Verification items for the finished model (mm, model axes). A direction names the side the tool comes from. Coordinates: 2 decimals unless noted, no trailing zeros. Order: outer loops, then holes, each group sorted by start corner. A loop starts at its lowest first (then second) coordinate and runs counter-clockwise, first axis right, second up. Notation, with made-up numbers: M -39.5,65.25 L -11.5,65.25 A6 ccw -11.5,73.25 Z; hole C 65,-16.75 d7. An arc over 180 degrees is marked long. Return JSON: item names as keys, results as strings. Group by question number.
Q1. Section check A-A, the plane y = -6. Enter the section's corners in (x, z).
Q2. Go/stop test with flat-tipped pins: pin 1 Ø10 at (x, z) = (-10, 34) entering from +Y; pin 2 Ø3.5 at (x, z) = (0.5, 36) entering from -Y; pin 3 Ø4 at (y, z) = (6.5, -3.5) entering from +X; pin 4 Ø12 at (x, y) = (-3, 18) entering from +Z. Record where each tip stops, or that it passes through.
Q3. Section check D-D, the plane z = 15. Enter the section's corners in (x, y), then the cut area to 3 significant figures.
Q4. Section check B-B, the plane x = 0. Enter the section's corners in (y, z), then the cut area to 3 significant figures.
Q5. Thickness scan on probe 1 along Z at (x, y) = (0, -3.5); probe 2 along X at (y, z) = (-8, 29.5); probe 3 along X at (y, z) = (-6, 39). Record the ranges inside material, lowest first.
Q6. Access from +Z, -Z, +X, -X, +Y, -Y to the whole of each face (thin tool, end or side, straight path). Record for faces 1 (the face through (0.71, -5.42, 52.99)), 2 (the face through (3.235, -5.862, 39.402)).
Q7. Section check C-C, the plane y = 16. Enter the section's corners in (x, z), then the cut area to 3 significant figures.
from build123d import *

# Parameters (mm, degrees)
F0_R     = 5.0192291216
F1_DEPTH = 11
F2_T     = -2.2
F3_R     = 7.6408252188
F4_DEPTH = 8
F5_R     = 6.0170563026
F6_DEPTH = 8.8
F7_DEPTH = 25


# Not quite as in the source:
# - a feature names something its author has since deleted; it is built from what else it names


with BuildPart() as f1:
    # F0 (on Front) → F1 (new body)
    with BuildSketch(Plane.XZ):
        with BuildLine():
            Line((6.7017039213, -13.6836004417), (7.7492278625, 17.3350542571))
            ThreePointArc((7.7492278625, 17.3350542571), (0.0056670875, 53.0044082442), (-7.7595389242, 17.3397601606))
            Line((-7.7595389242, 17.3397601606), (-6.7016295892, -13.6857909072))
            ThreePointArc((-6.7016295892, -13.6857909072), (-0.1142726876, -6.7527281229), (6.7055243621, -13.457278721))
            ThreePointArc((6.7055243621, -13.457278721), (6.7045691839, -13.570455703), (6.7017039213, -13.6836004417))
        make_face()
        with Locations((0, 34.3279652297)):
            Circle(F0_R, mode=Mode.SUBTRACT)
        with BuildLine():
            ThreePointArc((8.3308181793, 34.5567601339), (8.3292111279, 34.0466813329), (8.2964022532, 33.5376562417))
            Line((8.2964022532, 33.5376562417), (8.3308181793, 34.5567601339))
        make_face(mode=Mode.SUBTRACT)
        with BuildLine():
            ThreePointArc((-6.7016295892, -13.6857909072), (0.0010958632, -20.1628029936), (6.7017039213, -13.6836004417))
            ThreePointArc((6.7017039213, -13.6836004417), (6.7045691839, -13.570455703), (6.7055243621, -13.457278721))
            ThreePointArc((6.7055243621, -13.457278721), (-0.1142726876, -6.7527281229), (-6.7016295892, -13.6857909072))
        make_face()
        with BuildLine():
            Line((8.3308181793, 34.5567601339), (8.2964022532, 33.5376562417))
            ThreePointArc((8.2964022532, 33.5376562417), (8.3292111279, 34.0466813329), (8.3308181793, 34.5567601339))
        make_face()
        with Locations((0, 34.3279652297)):
            Circle(F0_R)
    extrude(amount=F1_DEPTH)

    # F2
    f2_openings = [f1.faces().sort_by_distance(p)[0] for p in [
        (-0.000731, -11, 23.334865),
    ]]
    offset(amount=F2_T, openings=f2_openings, kind=Kind.INTERSECTION)

    # F3 (on face) → F4 (join)
    with BuildSketch(Plane.XZ.offset(2.2)):
        with Locations((0, 34.3279652297)):
            Circle(F3_R)
    extrude(amount=F4_DEPTH)

    # F5 (on face) → F6 (cut)
    with BuildSketch(Plane.XZ.offset(10.2)):
        with Locations((0, 34.328058362)):
            Circle(F5_R)
    extrude(amount=-F6_DEPTH, mode=Mode.SUBTRACT)

    # F0 (on Front) → F7 (join)
    with BuildSketch(Plane.XZ):
        with BuildLine():
            ThreePointArc((-6.7016295892, -13.6857909072), (0.0010958632, -20.1628029936), (6.7017039213, -13.6836004417))
            ThreePointArc((6.7017039213, -13.6836004417), (6.7045691839, -13.570455703), (6.7055243621, -13.457278721))
            ThreePointArc((6.7055243621, -13.457278721), (-0.1142726876, -6.7527281229), (-6.7016295892, -13.6857909072))
        make_face()
    extrude(amount=-F7_DEPTH)


solid = f1.part
Numbers:
{
 "1": {"outline": "M -7.76,17.34 L -6.7,-13.69 A6.71 ccw 6.7,-13.68 L 7.75,17.34 A18.68 ccw long Z; C 0,34.33 d15.28; hole C 0,34.33 d12.03; hole M -5.61,18.84 L -4.5,-13.61 A4.51 ccw 4.5,-13.61 L 5.6,18.83 A16.48 ccw long Z"},
 "2": {"pin 1": "stops at y = 0", "pin 2": "stops at y = -1.4", "pin 3": "passes through", "pin 4": "stops at z = -6.75"},
 "3": {"outline": "M -7.68,-11 L -5.48,-11 L -5.48,-2.2 L 5.47,-2.2 L 5.47,-11 L 7.67,-11 L 7.67,0 L -7.68,0 Z", "area": "72.5 mm2"},
 "4": {"outline": "M -11,-20.16 L 25,-20.16 L 25,-6.75 L 0,-6.75 L 0,53 L -11,53 L -11,50.8 L -2.2,50.8 L -2.2,41.97 L -10.2,41.97 L -10.2,40.35 L -1.4,40.35 L -1.4,28.31 L -10.2,28.31 L -10.2,26.69 L -2.2,26.69 L -2.2,-17.96 L -11,-17.96 Z", "area": "551 mm2"},
 "5": {"probe 1": "z = -20.16 to -17.96, 26.69 to 28.31, 40.35 to 41.97, 50.8 to 53", "probe 2": "x = -18.04 to -15.75, -5.92 to -3.59, 3.59 to 5.92, 15.75 to 18.04", "probe 3": "x = -18.08 to -15.8, -6.05 to -3.79, 3.79 to 6.05, 15.8 to 18.08"},
 "6": {"face 1": "+Y, -Y", "face 2": "-Y"},
 "7": {"outline": "C 0,-13.46 d13.41", "area": "141 mm2"}
}
